Verification items for the finished model (mm, model axes). A direction names the side the tool comes from. Give positions to 0.01 mm unless a question says otherwise; leave off trailing zeros. Order: outer loops, then holes, each group sorted by start corner. A loop starts at its lowest first (then second) coordinate and runs counter-clockwise, first axis right, second up.
from build123d import *

# Parameters (mm, degrees)
SKETCH_1_W          = 130
SKETCH_1_H          = 100
EXTRUDE_1_DEPTH     = 25
SKETCH_2_W          = 50
SKETCH_2_H          = 50
SKETCH_2_R          = 10
EXTRUDE_2_DEPTH     = 100
SKETCH_3_R          = 11
CUT_EXTRUDE_1_DEPTH = 97.046863561
SKETCH_4_R          = 35.355339059
CUT_EXTRUDE_2_DEPTH = 35
SKETCH_5_W          = 45
SKETCH_5_H          = 25
CUT_EXTRUDE_3_DEPTH = 15


with BuildPart() as part:
    # Эскиз1 → Бобышка-Вытянуть1 (new body)
    with BuildSketch(Plane.XY):
        Rectangle(SKETCH_1_W, SKETCH_1_H)
    extrude(amount=EXTRUDE_1_DEPTH)

    # Эскиз2 → Бобышка-Вытянуть2 (add)
    with BuildSketch(Plane(origin=(0, 50, 0), x_dir=(1, 0, 0), z_dir=(0, 1, 0))):
        with Locations((0, -50)):
            Rectangle(SKETCH_2_W, SKETCH_2_H)
        with Locations(Location((0, -50, 0), (0, 0, 270))):
            Circle(SKETCH_2_R, mode=Mode.SUBTRACT)
    extrude(amount=-EXTRUDE_2_DEPTH)

    # Эскиз3 → Вырез-Вытянуть1 (cut, through all)
    with BuildSketch(Plane.XY.offset(25)):
        with Locations((48, 33)):
            Circle(SKETCH_3_R)
    extrude(amount=-CUT_EXTRUDE_1_DEPTH, mode=Mode.SUBTRACT)

    # Эскиз4 → Вырез-Вытянуть2 (cut, symmetric)
    with BuildSketch(Plane(origin=(0, 0, 0), x_dir=(-1, 0, 0), z_dir=(0, -1, 0))):
        with Locations((0, -50)):
            Circle(SKETCH_4_R)
    extrude(amount=CUT_EXTRUDE_2_DEPTH, both=True, mode=Mode.SUBTRACT)

    # Эскиз5 → Вырез-Вытянуть3 (cut)
    with BuildSketch(Plane.XY.offset(25)):
        with Locations((-42.5, 0)):
            Rectangle(SKETCH_5_W, SKETCH_5_H)
    extrude(amount=-CUT_EXTRUDE_3_DEPTH, mode=Mode.SUBTRACT)


solid = part.part
(1) Section check A-A, the plane x = 48. Enter the section's corners in (y, z).
Solved:
outline: (-50, 0) - (22, 0) - (22, 25) - (-50, 25) - close; (44, 0) - (50, 0) - (50, 25) - (44, 25) - close
(2) Section check D-D, the plane x = 0. Enter the section's corners in (y, z), then the cut area to 3 significant figures.
Solved:
outline: (-50, 0) - (50, 0) - (50, 40) - (35, 40) - (35, 14.64) - (-35, 14.64) - (-35, 40) - (-50, 40) - close; (-50, 60) - (-35, 60) - (-35, 75) - (-50, 75) - close; (35, 60) - (50, 60) - (50, 75) - (35, 75) - close
area: 2,680 mm2
(3) Section check C-C, the plane y = 33. Enter the section's corners in (x, z), then the cut area to 3 significant figures.
Solved:
outline: (-65, 0) - (37, 0) - (37, 25) - (25, 25) arc R35.36 cw to (-25, 25) - (-65, 25) - close; (59, 0) - (65, 0) - (65, 25) - (59, 25) - close
area: 2,340 mm2
(4) Set-up check for faces 1 (the flat face through (-25, 43, 50)), 2 (the flat face through (-43, 12.5, 18)), 3 (the flat face through (0, 35, 38)), 4 (the flat face through (45, 1, 25)): record each of +Z, -Z, +X, -X, +Y, -Y from which the full face is reachable in a straight line by a thin tool's end or side.
Solved:
face 1: +Z, -X, +Y, -Y
face 2: +Z, -X
face 3: +Z
face 4: +Z, +X, +Y, -Y
(5) Scan lines: line 1 (Y direction, x = 24.5, z = 54); line 2 (X direction, y = 41, z = 50); line 3 (Z direction, x = 34.5, y = 10). Record each from-to range of solid material in increasing order.
Solved:
line 1: y = -50 to -35, 35 to 50
line 2: x = -25 to -10, 10 to 25
line 3: z = 0 to 25
(6) Go/stop test with flat-tipped pins: pin 1 (16.5 mm diameter, centred on y = 44.5, z = 54.5, fed in from +X); pin 2 (12.5 mm diameter, centred on x = -45, y = -4, fed in from +Z); pin 3 (6 mm diameter, centred on y = -31, z = 59.5, fed in from -X); pin 4 (12 mm diameter, centred on y = 40.5, z = 61.5, fed in from -X). Record where each tip stops, or that it passes through.
Solved:
pin 1: stops at x = 25
pin 2: stops at z = 10
pin 3: passes through
pin 4: stops at x = -25
(7) Release check for a two-part mould opening along Y. For faces 5 (the flat face through (0, -35, 38)), 6 (the flat face through (-1, 50, 29)), 7 (the flat face through (-45, -31, 25)) record: pulls with the +Y half, pulls with the -Y half, needs draft (parallel to the pull), parting line crosses it, or undercut.
Solved:
face 5: undercut
face 6: pulls with the +Y half
face 7: needs draft
(8) Section check B-B, the plane z = 50. Enter the section's corners in (x, y).
Solved:
outline: (-25, -50) - (-10, -50) - (-10, -35) - (-25, -35) - close; (-25, 35) - (-10, 35) - (-10, 50) - (-25, 50) - close; (10, -50) - (25, -50) - (25, -35) - (10, -35) - close; (10, 35) - (25, 35) - (25, 50) - (10, 50) - close
